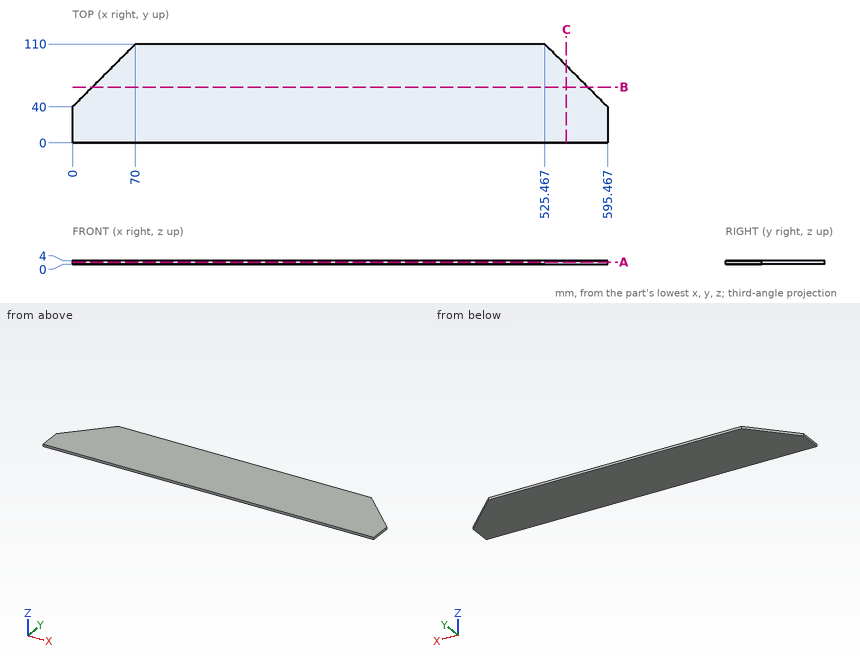
Part print with two shaded views. Sizes in mm from the minimum x, y, z corner. Give positions to 0.01 mm unless a question says otherwise; leave off trailing zeros. Order: outer loops, then holes, each group sorted by start corner. A loop starts at its lowest first (then second) coordinate and runs counter-clockwise, first axis right, second up. Notation, with made-up numbers: (64, -9) - (80, -9) arc R22 cw to (80, 23) - close; hole circle Ø5 at (47.25, -17.5). An arc over 180 degrees is marked (long way). Write each question's results on one line, items separated by ' | '.
1. Saw through at B-B on y = 62. List the corners of the cut face in (x, z).
Calculated:
outline: (22, 0) - (573.47, 0) - (573.47, 4) - (22, 4) - close
2. Pin check, flat tip, straight feed: pin 1 (10 mm diameter, centred on x = 363, y = 33.5, fed in from -Z). Stop position of the tip, or through.
Calculated:
pin 1: stops at z = 0
3. Probe L1, parallel to Y at x = 551, z = 0.55 (1 decimal); L2, parallel to X at y = 57, z = 0.7 (1 decimal); L3, parallel to X at y = 59, z = 3 (1 decimal). List the from-to ranges inside material, lowest first. Write a range as from..to.
Calculated:
L1: y = 0..84.5 | L2: x = 17..578.5 | L3: x = 19..576.5
4. Saw through at A-A on z = 2.5. List the corners of the cut face in (x, y).
Calculated:
outline: (0, 0) - (595.47, 0) - (595.47, 40) - (525.47, 110) - (70, 110) - (0, 40) - close
5. Saw through at C-C on x = 549.5. List the corners of the cut face in (y, z), and give its area (3 significant figures).
Calculated:
outline: (0, 0) - (85.97, 0) - (85.97, 4) - (0, 4) - close | area: 344 mm2
